from build123d import *

# Parameters (mm, degrees)
ESTRUSIONE_SOTTILE1_DEPTH = 6
RACCORDO3_R               = 6
SCHIZZO4_R                = 2
TAGLIO_ESTRUSIONE1_DEPTH  = 0.75
TAGLIO_ESTRUSIONE2_DEPTH  = 0.75
RACCORDO1_R               = 0.75
RACCORDO2_R               = 0.5


with BuildPart() as part:
    # Schizzo1 → Estrusione-Sottile1 (new, symmetric)
    with BuildSketch(Plane.XY):
        Polygon((9.192388155, 9.192388155), (0, 0), (-11, 0), (-11, 0.75), (-0.310660172, 0.75), (8.66205807, 9.722718241), align=None)
    extrude(amount=ESTRUSIONE_SOTTILE1_DEPTH, both=True)

    # Raccordo3
    raccordo3_edges = [part.edges().sort_by_distance(p)[0] for p in [
        (-11, 0.375, 6),
        (-11, 0.375, -6),
        (8.927223112, 9.457553198, -6),
        (8.927223112, 9.457553198, 6),
    ]]
    fillet(raccordo3_edges, radius=RACCORDO3_R - 0.0001)  # a hair under: the kernel refuses the full size

    # Schizzo4 → Taglio-Estrusione1 (cut)
    with BuildSketch(Plane(origin=(0, 0.75, 0), x_dir=(1, 0, 0), z_dir=(0, 1, 0))):
        with Locations(Location((-7, 0, 0), (0, 0, 180))):
            Circle(SCHIZZO4_R)
    extrude(amount=-TAGLIO_ESTRUSIONE1_DEPTH, mode=Mode.SUBTRACT)

    # Schizzo5 → Taglio-Estrusione2 (cut)
    with BuildSketch(Plane(origin=(-0.530330086, 0.530330086, 0), x_dir=(0, 0, 1), z_dir=(-0.7071067811865491, 0.7071067811865459, 0))):
        with BuildLine():
            Line((2, 9), (2, 3.5))
            ThreePointArc((2, 3.5), (0, 1.5), (-2, 3.5))
            Line((-2, 3.5), (-2, 9))
            ThreePointArc((-2, 9), (0, 11), (2, 9))
        make_face()
    extrude(amount=-TAGLIO_ESTRUSIONE2_DEPTH, mode=Mode.SUBTRACT)

    # Raccordo1
    raccordo1_edges = [part.edges().sort_by_distance(p)[0] for p in [
        (0, 0, 0),
    ]]
    fillet(raccordo1_edges, radius=RACCORDO1_R)

    # Raccordo2
    raccordo2_edges = [part.edges().sort_by_distance(p)[0] for p in [
        (-0.310660172, 0.75, 0),
    ]]
    fillet(raccordo2_edges, radius=RACCORDO2_R)


solid = part.part
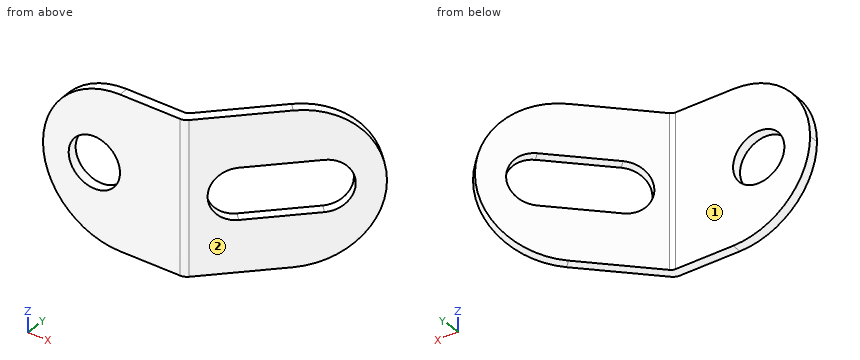
Can you work these out from the model? Positions are in its coordinate system, mm. Face numbers are marked on the shaded views. A direction names the side the tool comes from. Round coordinates to 2 decimals unless told otherwise and drop trailing zeros. Write each loop counter-clockwise with the first axis right and the second up, starting at its lowest first coordinate (ties: lowest second). Pieces come first, ordered by that corner, then holes. Notation, with made-up numbers: (-33.5, 50.5) -> (-9.5, 50.5) arc R19 ccw to (-9.5, 65.5) -> close; hole circle Ø4 at (5.5, -3.5). An arc over 180 degrees is marked (long way). Use one line per item in the form item = value. Start each with the question number.
Q1. If I drill on probe 1 along Y at (x, z) = (-5.25, 4); probe 2 along Z at (x, y) = (-7, 0.25); probe 3 along X at (y, z) = (2.5, -3.5), over which ranges is the centre line in solid material (lowest first)? Write a range as [from, to].
Q2. Imagine slicing it at C-C (z = -1). Please give me the cut outline in (x, y).
Q3. Imagine slicing it at D-D (z = 4.25). Please give me the cut outline in (x, y), then the cut area to 3 significant figures.
Q4. Which directions (+Z, -Z, +X, -X, +Y, -Y) give clear straight access to the entire face, cutting with the end or side of a thin tool? Please do the marked faces 1 and 2.
Q5. Imagine slicing it at B-B (y = 4.5). Please give me the cut outline in (x, z).
Q6. Imagine slicing it at A-A (x = -7.5). Please give me the cut outline in (y, z), then the cut area to 3 significant figures.
Q7. I'm going to push flat-ended pins straight in: P1, Ø3, axis at x = -4.5, z = -2, coming from the +Y side; P2, Ø1.5, axis at x = -7.5, z = 1, coming from the -Y side; P3, Ø2, axis at x = 6.5, z = -2.5, coming from the +Y side; P4, Ø2, axis at y = 1, z = 4.5, coming from the -X side. Where does each tip first touch, or does it pass through?
Worked out:
q1.probe_1 = [0, 0.75]
q1.probe_2 = [-5.66, -2], [2, 5.66]
q1.probe_3 = [1.44, 2.5]
q2.outline = (-10.92, 0) -> (-8.73, 0) -> (-8.73, 0.75) -> (-10.92, 0.75) -> close; (-5.27, 0) -> (-0.31, 0) arc R0.75 ccw to (0.22, 0.22) -> (1.25, 1.25) -> (0.72, 1.78) -> (-0.16, 0.9) arc R0.5 cw to (-0.52, 0.75) -> (-5.27, 0.75) -> close; (7.06, 8.12) -> (7.59, 7.59) -> (9.13, 9.13) -> (8.6, 9.66) -> close
q3.outline = (-9.24, 0) -> (-0.31, 0) arc R0.75 ccw to (0.22, 0.22) -> (7.94, 7.94) -> (7.41, 8.47) -> (-0.16, 0.9) arc R0.5 cw to (-0.52, 0.75) -> (-9.24, 0.75) -> close
q3.area = 15.1 mm^2
q4.face_1 = +Z, -Z, -X, +Y
q4.face_2 = +Z, -Z, +X, -Y
q5.outline = (3.44, -6) -> (4.5, -6) -> (4.5, -2) -> (3.44, -2) -> close; (3.44, 2) -> (4.5, 2) -> (4.5, 6) -> (3.44, 6) -> close
q6.outline = (0, -5.45) -> (0.75, -5.45) -> (0.75, -1.94) -> (0, -1.94) -> close; (0, 1.94) -> (0.75, 1.94) -> (0.75, 5.45) -> (0, 5.45) -> close
q6.area = 5.28 mm^2
q7.P1 = 0.75
q7.P2 = through
q7.P3 = 8.56
q7.P4 = -9.85
